from build123d import *

# Parameters (mm, degrees)
SKETCH1_R           = 25
BOSS_EXTRUDE1_DEPTH = 300
SHELL1_T            = -5
FILLET1_R           = 5
SKETCH2_W           = 30
SKETCH2_H           = 25
BOSS_EXTRUDE2_DEPTH = 40
SKETCH3_R           = 10
CUT_EXTRUDE1_DEPTH  = 40
FILLET3_R           = 15


with BuildPart() as part:
    # Sketch1 → Boss-Extrude1 (new body)
    with BuildSketch(Plane(origin=(0, 0, 0), x_dir=(1, 0, 0), z_dir=(0, 1, 0))):
        with Locations(Location((0, 0, 0), (0, 0, 270))):
            Circle(SKETCH1_R)
    extrude(amount=BOSS_EXTRUDE1_DEPTH)

    # Shell1
    shell1_openings = [part.faces().sort_by_distance(p)[0] for p in [
        (0, 300, 0),
    ]]
    offset(amount=SHELL1_T, openings=shell1_openings, kind=Kind.INTERSECTION)

    # Fillet1
    fillet1_edges = [part.edges().sort_by_distance(p)[0] for p in [
        (0, 0, -25),
    ]]
    fillet(fillet1_edges, radius=FILLET1_R)

    # Sketch2 → Boss-Extrude2 (add)
    with BuildSketch(Plane.XZ):
        Rectangle(SKETCH2_W, SKETCH2_H)
    extrude(amount=BOSS_EXTRUDE2_DEPTH)

    # Sketch3 → Cut-Extrude1 (cut)
    with BuildSketch(Plane(origin=(0, 0, -12.5), x_dir=(-1, 0, 0), z_dir=(0, 0, -1))):
        with Locations((0, -25)):
            Circle(SKETCH3_R)
    extrude(amount=-CUT_EXTRUDE1_DEPTH, mode=Mode.SUBTRACT)

    # Fillet3
    fillet3_edges = [part.edges().sort_by_distance(p)[0] for p in [
        (-15, -40, 0),
        (15, -40, 0),
    ]]
    fillet(fillet3_edges, radius=FILLET3_R - 0.0001)  # a hair under: the kernel refuses the full size


solid = part.part
Could you check a few things on this model? Use its own coordinates, in mm. A direction names the side the tool comes from. Give positions to 0.01 mm unless a question says otherwise; leave off trailing zeros. Order: outer loops, then holes, each group sorted by start corner. A loop starts at its lowest first (then second) coordinate and runs counter-clockwise, first axis right, second up. Notation, with made-up numbers: (-9.75, 70.25) - (-4.75, 70.25) arc R19 cw to (-4.75, 98.25) - close; hole circle Ø7 at (-11.75, 6). An arc over 180 degrees is marked (long way). One line per question, with ' | ' between items. Start each with the question number.
Item 1: Thinking about a two-plate mould opening in X: for faces 1 (the cylindrical face through (7.509, 150.435, 23.846)), 2 (the cylindrical face through (-5.38, -16.57, -0.18)), 3 (the flat face through (-15, -12, 0)), 4 (the cylindrical face through (10.72, -35.49, 0.18)), which applies, pulls with the +X half, pulls with the -X half, needs draft (parallel to the pull), parting line crosses it, or undercut?
Item 2: I'm going to push flat-ended pins straight in: pin 1 Ø1.5 at (y, z) = (5, 15) entering from +X; pin 2 Ø8 at (x, y) = (8.5, 166) entering from -Z; pin 3 Ø9 at (x, y) = (5, -15) entering from -Z. Where does each tip first touch, or does it pass through?
Item 3: I need wall thicknesses on probe 1 along Y at (x, z) = (0, 1); probe 2 along X at (y, z) = (195, 0); probe 3 along Z at (x, y) = (12, 22). Which ranges of each line are inside material? Lowest first, please. Write a range as [from, to].
Item 4: I want a section at A-A on y = 144.5. Write out the boundary of the cut face in (x, z), then the cut area to 3 significant figures.
Item 5: For faces 5 (the cylindrical face through (-10.72, -35.49, 0.18)), 6 (the flat face through (15, -12, 0)), 7 (the flat face through (-4, -15, -12.5)), 8 (the cylindrical face through (-19.524, 150.435, -4.336)), 9 (the flat face through (-4, -15, 12.5)), which set-ups out of +Z, -Z, +X, -X, +Y, -Y let a thin tool reach every point of the face, with its end or its side?
Verdict:
1) face 1: parting line crosses it | face 2: undercut | face 3: pulls with the -X half | face 4: pulls with the +X half
2) pin 1: x = 20.54 | pin 2: z = -24.59 | pin 3: z = -12.5
3) probe 1: [-40, -35], [-15, 5] | probe 2: [-25, -20], [20, 25] | probe 3: [-21.93, -16], [16, 21.93]
4) outline: circle Ø50 at (0, 0); hole circle Ø40 at (0, 0) | area: 707 mm^2
5) face 5: +Z, -Z, -X, -Y | face 6: +Z, -Z, +X, -Y | face 7: -Z, +X, -X, -Y | face 8: +Y | face 9: +Z, +X, -X, -Y
